```python
from build123d import *

# Parameters (mm, degrees)
BOSS_EXTRUDE1_DEPTH      = 19
BOSS_EXTRUDE2_DEPTH      = 7.5
BOSS_EXTRUDE3_DEPTH      = 7.5
CUT_EXTRUDE1_DEPTH       = 6.5
FILLET2_R                = 5
FILLET3_R                = 5
FILLET4_R                = 1
SKETCH3_R                = 7
BOSS_EXTRUDE4_DEPTH      = 20
BOSS_EXTRUDE4_DEPTH_BACK = 18


with BuildPart() as part:
    # Sketch1 → Boss-Extrude1 (new body)
    with BuildSketch(Plane(origin=(0, 0, 0), x_dir=(0, 0, -1), z_dir=(1, 0, 0))):
        with BuildLine():
            ThreePointArc((32, 0), (0, 32), (-32, 0))
            Line((-32, 0), (-31, 0))
            ThreePointArc((-31, 0), (0, 31), (31, 0))
            Line((31, 0), (32, 0))
        make_face()
    extrude(amount=BOSS_EXTRUDE1_DEPTH)

    # Sketch1_3 → Boss-Extrude2 (add)
    with BuildSketch(Plane(origin=(0, 0, 0), x_dir=(0, 0, -1), z_dir=(1, 0, 0))):
        with BuildLine():
            ThreePointArc((31, 0), (0, 31), (-31, 0))
            Line((-31, 0), (31, 0))
        make_face()
    extrude(amount=BOSS_EXTRUDE2_DEPTH)

    # Sketch2 → Boss-Extrude3 (add)
    with BuildSketch(Plane(origin=(7.5, 0, 0), x_dir=(0, 0, -1), z_dir=(1, 0, 0))):
        with BuildLine():
            Line((6.5, 0), (5, 0))
            ThreePointArc((5, 0), (0, -5), (-5, 0))
            Line((-5, 0), (-6.5, 0))
            Line((-6.5, 0), (-6.5, -5.529275222))
            Line((-6.5, -5.529275222), (6.5, -5.529275222))
            Line((6.5, -5.529275222), (6.5, 0))
        make_face()
        with BuildLine():
            ThreePointArc((-5, 0), (0, -5), (5, 0))
            Line((5, 0), (-5, 0))
        make_face()
        with BuildLine():
            Line((-5, 0), (5, 0))
            ThreePointArc((5, 0), (0, 5), (-5, 0))
        make_face()
    extrude(amount=-BOSS_EXTRUDE3_DEPTH)

    # Sketch2_3 → Cut-Extrude1 (cut)
    with BuildSketch(Plane(origin=(7.5, 0, 0), x_dir=(0, 0, -1), z_dir=(1, 0, 0))):
        with BuildLine():
            ThreePointArc((-5, 0), (0, -5), (5, 0))
            Line((5, 0), (-5, 0))
        make_face()
        with BuildLine():
            Line((-5, 0), (5, 0))
            ThreePointArc((5, 0), (0, 5), (-5, 0))
        make_face()
    extrude(amount=-CUT_EXTRUDE1_DEPTH, mode=Mode.SUBTRACT)

    # Mirror2: part across plane


with BuildPart() as part_1:
    add(part.part)
    add(part.part.mirror(Plane(origin=(0, 0, 0), x_dir=(0, 0, 1), z_dir=(1, 0, 0))))

    # Fillet2
    fillet2_edges = [part_1.edges().sort_by_distance(p)[0] for p in [
        (0, 0, -6.5),
    ]]
    fillet(fillet2_edges, radius=FILLET2_R)

    # Fillet3
    fillet3_edges = [part_1.edges().sort_by_distance(p)[0] for p in [
        (0, 0, 6.5),
    ]]
    fillet(fillet3_edges, radius=FILLET3_R)

    # Fillet4
    fillet4_edges = [part_1.edges().sort_by_distance(p)[0] for p in [
        (0, -5.529275222, 6.5),
        (0, -5.529275222, -6.5),
    ]]
    fillet(fillet4_edges, radius=FILLET4_R)

    # Sketch3 → Boss-Extrude4 (add, two sides)
    with BuildSketch(Plane(origin=(0, 32, 0), x_dir=(1, 0, 0), z_dir=(0, 1, 0))) as boss_extrude4_sk:
        with Locations((0, -21.25)):
            Circle(SKETCH3_R)
    extrude(amount=BOSS_EXTRUDE4_DEPTH)
    extrude(boss_extrude4_sk.sketch, amount=-BOSS_EXTRUDE4_DEPTH_BACK)


solid = part_1.part
```
Design review of the part built by this model. Coordinates are the model's own, in mm. A direction names the side the tool comes from. Coordinates: 2 decimals unless noted, no trailing zeros. Write each loop counter-clockwise with the first axis right and the second up, starting at its lowest first coordinate (ties: lowest second). Pieces come first, ordered by that corner, then holes.
1) Insertion check: pin 1 (11 mm diameter, centred on y = -1.5, z = -1, fed in from +X); pin 2 (8 mm diameter, centred on y = 8.5, z = 17, fed in from -X); pin 3 (6 mm diameter, centred on x = 0, z = -23, fed in from -Y); pin 4 (12 mm diameter, centred on x = -7, y = 5, fed in from -Z). Each pin has a flat end and moves straight along its axis. Give the tip position at first contact, or say it passes through.
2) Add section A-A (z = -8). Write out the cut boundary in (x, y), plus the area to 3 significant figures.
3) Add section B-B (y = 22.5). Write out the cut boundary in (x, z), plus the area to 3 significant figures.
4) To check wall thickness, follow L1, parallel to Y at x = 3.75, z = 0; L2, parallel to Z at x = 12.5, y = 21; L3, parallel to X at y = 3.5, z = 18.5. State the ranges of each line that lie inside material, in increasing order.
5) Mouldability with a two-part tool opening along Y and no side actions: class faces 1 (the cylindrical face through (4.3, -4.88, 1.08)), 2 (the flat face through (-19, 31.5, 0.1)), 3 (the cylindrical face through (0.266, 31.992, -0.704)) as +Y half, -Y half, draft (parallel to the pull), parting line (faces both ways), or undercut.
6) Add section C-C (x = -14). Write out the cut boundary in (y, z).
7) Machinability: for faces 4 (the flat face through (7.5, 13, 0)), 5 (the cylindrical face through (-1.517, 37.876, 28.084)), 6 (the flat face through (1, 0, 0)), 7 (the cylindrical face through (-13.17, 30.993, 0.682)), which of the approach directions +Z, -Z, +X, -X, +Y, -Y give a long, thin tool a straight path to every point of the face, cutting with its end or side? Answer none if there is none.
8) Add section D-D (z = 17.5). Write out the cut boundary in (x, y).
Check result:
1. pin 1: stops at x = 7.5
1. pin 2: stops at x = -7.5
1. pin 3: stops at y = 0
1. pin 4: stops at z = -32
2. outline: (-19, 29.95) - (-7.5, 29.95) - (-7.5, -1.43) - (7.5, -1.43) - (7.5, 29.95) - (19, 29.95) - (19, 30.98) - (-19, 30.98) - close
2. area: 510 mm2
3. outline: (-19, -22.75) - (19, -22.75) - (19, -21.32) - (7.5, -21.32) - (7.5, 21.32) - (19, 21.32) - (19, 22.75) - (6.84, 22.75) arc R7 ccw to (-6.84, 22.75) - (-19, 22.75) - (-19, 21.32) - (-7.5, 21.32) - (-7.5, -21.32) - (-19, -21.32) - close
3. area: 804 mm2
4. L1: y = -5.53 to -5, 5 to 32
4. L2: z = -24.15 to -22.8, 22.8 to 24.15
4. L3: x = -7.5 to 7.5
5. face 1: undercut
5. face 2: draft
5. face 3: +Y half
6. outline: (0, -32) arc R32 ccw to (0, 32) - (0, 31) arc R31 cw to (0, -31) - close
7. face 4: +X, -Y
7. face 5: +Y
7. face 6: +X
7. face 7: -X, -Y
8. outline: (-19, 25.59) - (-7.5, 25.59) - (-7.5, 0) - (7.5, 0) - (7.5, 25.59) - (19, 25.59) - (19, 26.79) - (5.91, 26.79) - (5.91, 52) - (-5.91, 52) - (-5.91, 26.79) - (-19, 26.79) - close
